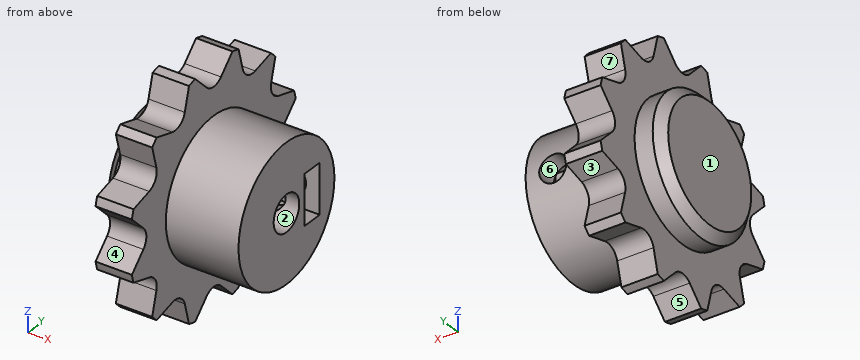
```python
from build123d import *

# Parameters (mm, degrees)
F0_R          = 7.5
F0_R_2        = 2
F1_DEPTH      = 12
F1_DEPTH_BACK = 3
F2_DEPTH      = 4
F3_DEPTH      = 3
F4_SIZE       = 1
F5_W          = 2.4
F5_H          = 5.5
F6_DEPTH      = 7
F7_R          = 1.5
F8_DEPTH      = 10.0078377589
F8_DEPTH_BACK = 1.4781244445


with BuildPart() as f1:
    # F0 (on Right) → F1 (new body, two sides)
    with BuildSketch(Plane.YZ) as f1_sk:
        Circle(F0_R)
        Circle(F0_R_2, mode=Mode.SUBTRACT)
    extrude(amount=F1_DEPTH)
    extrude(f1_sk.sketch, amount=-F1_DEPTH_BACK)

    # F0 (on Right) → F2 (join)
    with BuildSketch(Plane.YZ):
        with BuildLine():
            Line((-1.1225320151, 11.0123179849), (-2.9170517891, 12.8068377589))
            ThreePointArc((-2.9170517891, 12.8068377589), (-3.3995493346, 12.6872908394), (-3.8771779259, 12.5495727359))
            Line((-3.8771779259, 12.5495727359), (-4.5340177508, 10.098213137))
            ThreePointArc((-4.5340177508, 10.098213137), (-5.273675, 9.1342730426), (-6.4783002341, 8.9756811219))
            Line((-6.4783002341, 8.9756811219), (-8.929659833, 9.6325209468))
            ThreePointArc((-8.929659833, 9.6325209468), (-9.2877415049, 9.2877415049), (-9.6325209468, 8.929659833))
            Line((-9.6325209468, 8.929659833), (-8.9756811219, 6.4783002341))
            ThreePointArc((-8.9756811219, 6.4783002341), (-9.1342730426, 5.273675), (-10.098213137, 4.5340177508))
            Line((-10.098213137, 4.5340177508), (-12.5495727359, 3.8771779259))
            ThreePointArc((-12.5495727359, 3.8771779259), (-12.6872908394, 3.3995493346), (-12.8068377589, 2.9170517891))
            Line((-12.8068377589, 2.9170517891), (-11.0123179849, 1.1225320151))
            ThreePointArc((-11.0123179849, 1.1225320151), (-10.54735, 0), (-11.0123179849, -1.1225320151))
            Line((-11.0123179849, -1.1225320151), (-12.8068377589, -2.9170517891))
            ThreePointArc((-12.8068377589, -2.9170517891), (-12.6872908394, -3.3995493346), (-12.5495727359, -3.8771779259))
            Line((-12.5495727359, -3.8771779259), (-10.098213137, -4.5340177508))
            ThreePointArc((-10.098213137, -4.5340177508), (-9.1342730426, -5.273675), (-8.9756811219, -6.4783002341))
            Line((-8.9756811219, -6.4783002341), (-9.6325209468, -8.929659833))
            ThreePointArc((-9.6325209468, -8.929659833), (-9.2877415049, -9.2877415049), (-8.929659833, -9.6325209468))
            Line((-8.929659833, -9.6325209468), (-6.4783002341, -8.9756811219))
            ThreePointArc((-6.4783002341, -8.9756811219), (-5.273675, -9.1342730426), (-4.5340177508, -10.098213137))
            Line((-4.5340177508, -10.098213137), (-3.8771779259, -12.5495727359))
            ThreePointArc((-3.8771779259, -12.5495727359), (-3.3995493346, -12.6872908394), (-2.9170517891, -12.8068377589))
            Line((-2.9170517891, -12.8068377589), (-1.1225320151, -11.0123179849))
            ThreePointArc((-1.1225320151, -11.0123179849), (0, -10.54735), (1.1225320151, -11.0123179849))
            Line((1.1225320151, -11.0123179849), (2.9170517891, -12.8068377589))
            ThreePointArc((2.9170517891, -12.8068377589), (3.3995493346, -12.6872908394), (3.8771779259, -12.5495727359))
            Line((3.8771779259, -12.5495727359), (4.5340177508, -10.098213137))
            ThreePointArc((4.5340177508, -10.098213137), (5.273675, -9.1342730426), (6.4783002341, -8.9756811219))
            Line((6.4783002341, -8.9756811219), (8.929659833, -9.6325209468))
            ThreePointArc((8.929659833, -9.6325209468), (9.2877415049, -9.2877415049), (9.6325209468, -8.929659833))
            Line((9.6325209468, -8.929659833), (8.9756811219, -6.4783002341))
            ThreePointArc((8.9756811219, -6.4783002341), (9.1342730426, -5.273675), (10.098213137, -4.5340177508))
            Line((10.098213137, -4.5340177508), (12.5495727359, -3.8771779259))
            ThreePointArc((12.5495727359, -3.8771779259), (12.6872908394, -3.3995493346), (12.8068377589, -2.9170517891))
            Line((12.8068377589, -2.9170517891), (11.0123179849, -1.1225320151))
            ThreePointArc((11.0123179849, -1.1225320151), (10.54735, 0), (11.0123179849, 1.1225320151))
            Line((11.0123179849, 1.1225320151), (12.8068377589, 2.9170517891))
            ThreePointArc((12.8068377589, 2.9170517891), (12.6872908394, 3.3995493346), (12.5495727359, 3.8771779259))
            Line((12.5495727359, 3.8771779259), (10.098213137, 4.5340177508))
            ThreePointArc((10.098213137, 4.5340177508), (9.1342730426, 5.273675), (8.9756811219, 6.4783002341))
            Line((8.9756811219, 6.4783002341), (9.6325209468, 8.929659833))
            ThreePointArc((9.6325209468, 8.929659833), (9.2877415049, 9.2877415049), (8.929659833, 9.6325209468))
            Line((8.929659833, 9.6325209468), (6.4783002341, 8.9756811219))
            ThreePointArc((6.4783002341, 8.9756811219), (5.273675, 9.1342730426), (4.5340177508, 10.098213137))
            Line((4.5340177508, 10.098213137), (3.8771779259, 12.5495727359))
            ThreePointArc((3.8771779259, 12.5495727359), (3.3995493346, 12.6872908394), (2.9170517891, 12.8068377589))
            Line((2.9170517891, 12.8068377589), (1.1225320151, 11.0123179849))
            ThreePointArc((1.1225320151, 11.0123179849), (0, 10.54735), (-1.1225320151, 11.0123179849))
        make_face()
        Circle(F0_R, mode=Mode.SUBTRACT)
        Circle(F0_R_2)
    extrude(amount=F2_DEPTH)

    # F3 (add): a face of the model
    f3_faces = [f1.faces().sort_by_distance(p)[0] for p in [
        (0, 0, 0),
    ]]
    extrude(f3_faces, amount=F3_DEPTH)

    # F4
    f4_edges = [f1.edges().sort_by_distance(p)[0] for p in [
        (-3, -7.5, 0),
    ]]
    chamfer(f4_edges, length=F4_SIZE)

    # F5 (on face) → F6 (cut)
    with BuildSketch(Plane.YZ.offset(12)):
        with Locations((4, 0)):
            Rectangle(F5_W, F5_H)
    extrude(amount=-F6_DEPTH, mode=Mode.SUBTRACT)

    # F7 (on face) → F8 (cut, two sides)
    with BuildSketch(Plane(origin=(0, 2.8, 0), x_dir=(-1, 0, 0), z_dir=(0, 1, 0))) as f8_sk:
        with Locations((-9, 0)):
            Circle(F7_R)
    extrude(amount=F8_DEPTH, mode=Mode.SUBTRACT)
    extrude(f8_sk.sketch, amount=-F8_DEPTH_BACK, mode=Mode.SUBTRACT)


solid = f1.part
```
The model under review builds one solid part; all positions refer to its coordinate system, in mm. Face numbers are marked on the shaded views. A direction names the side the tool comes from. Round coordinates to 2 decimals unless told otherwise and drop trailing zeros. Loops run counter-clockwise (first coordinate to the right, second up) from the corner with the lowest first, then second, coordinate; pieces in that order, holes last.
Item 1: Take a section at D-D (x = 9). Write out the cut boundary in (y, z).
Determined:
outline: (1.32, -1.5) arc R2 cw (long way) to (1.32, 1.5) - (2.8, 1.5) - (2.8, 2.75) - (5.2, 2.75) - (5.2, 1.5) - (7.35, 1.5) arc R7.5 ccw (long way) to (7.35, -1.5) - (5.2, -1.5) - (5.2, -2.75) - (2.8, -2.75) - (2.8, -1.5) - close
Item 2: Take a section at B-B (y = 0). Write out the cut boundary in (x, z), then the cut area to 3 significant figures.
Determined:
outline: (-3, -6.5) - (-2, -7.5) - (0, -7.5) - (0, -10.55) - (4, -10.55) - (4, -7.5) - (12, -7.5) - (12, -2) - (4, -2) - (4, 2) - (12, 2) - (12, 7.5) - (4, 7.5) - (4, 10.55) - (0, 10.55) - (0, 7.5) - (-2, 7.5) - (-3, 6.5) - close
area: 216 mm2
Item 3: Take a section at C-C (x = 6.75). Write out the cut boundary in (y, z), then the cut area to 3 significant figures.
Determined:
outline: circle Ø15 at (0, 0); hole circle Ø4 at (0, 0); hole (2.8, -2.75) - (5.2, -2.75) - (5.2, 2.75) - (2.8, 2.75) - close
area: 151 mm2
Item 4: Take a section at A-A (z = 0). Give the number of separate pieces and of enclosed holes in the cut face, then the cut area to 3 significant figures.
Determined:
separate pieces: 3
enclosed holes: 0
area: 190 mm2
Item 5: Mouldability with a two-part tool opening along Z and no side actions: class the marked faces 1, 2 and 3 as released by +Z, released by -Z, zero draft, split by the parting line, or undercut.
Determined:
face 1: zero draft
face 2: undercut
face 3: released by -Z
Item 6: For the marked faces 4, 5, 6 and 7, list the 3-axis set-ups (+Z, -Z, +X, -X, +Y, -Y) from which the entire face can be reached by the end or side of a thin tool; tool diameter is ignored.
Determined:
face 4: +X, -X, -Y
face 5: -Z, +X, -X
face 6: +Y
face 7: +X, -X, +Y
Item 7: For line 1 (Z direction, x = 7.75, y = 0); line 2 (X direction, y = 2.3, z = 0); line 3 (Y direction, x = 8.5, z = -1.5), list the stretches that pass through material, from the lowest coordinate up.
Determined:
line 1: z = -7.5 to -2, 2 to 7.5
line 2: x = -3 to 7.5, 10.5 to 12
line 3: y = -7.35 to -1.32, 1.32 to 2.8, 5.2 to 7.35
Item 8: Clearance check with flat-ended pins moving along their axes: pin 1 Ø4 at (y, z) = (8, 8.5) entering from +X; pin 2 Ø0.7 at (x, y) = (7.5, 4) entering from -Z; pin 3 Ø4.5 at (x, z) = (7, 0.5) entering from -Y. State where each tip first meets the part, or that it passes through.
Determined:
pin 1: stops at x = 4
pin 2: stops at z = -6.55
pin 3: stops at y = -7.5
